```python
from build123d import *

# Parameters (mm, degrees)
BASE_FLANGE1_DEPTH           = 1
EDGE_FLANGE1_STRIP_W         = 8
EDGE_FLANGE1_STRIP_H         = 1
EDGE_FLANGE1_STRIP_CUT_DEPTH = 24
EDGE_FLANGE1_DEPTH           = 24
HEM1_START                   = -12
HEM1_DEPTH                   = 24
HEM1_2_DEPTH                 = 24
CUT_EXTRUDE1_DEPTH           = 10


# Read off the part's stored shape, not the designer's step: Hem1
# Sheet-metal steps are written as plain solids
with BuildPart() as part:
    # Sketch1 → Base-Flange1 (new body)
    with BuildSketch(Plane(origin=(0, 0, 0), x_dir=(1, 0, 0), z_dir=(0, 1, 0))):
        with BuildLine():
            Line((-5.5, 12), (5.5, 12))
            Line((5.5, 12), (18.155635881, 7.546363234))
            ThreePointArc((18.155635881, 7.546363234), (23.5, 0), (18.155635881, -7.546363234))
            Line((18.155635881, -7.546363234), (5.5, -12))
            Line((5.5, -12), (-5.5, -12))
            Line((-5.5, -12), (-5.5, 12))
        make_face()
        with BuildLine():
            Line((10.34, 2.38), (13.012470906, 2.38))
            ThreePointArc((13.012470906, 2.38), (18.942702571, 0), (13.012470906, -2.38))
            Line((13.012470906, -2.38), (10.34, -2.38))
            ThreePointArc((10.34, -2.38), (7.96, 0), (10.34, 2.38))
        make_face(mode=Mode.SUBTRACT)
    extrude(amount=BASE_FLANGE1_DEPTH)

    # Edge-Flange1 strip (across the edge) → Edge-Flange1 strip cut (cut)
    with BuildSketch(Plane(origin=(-5.5, 1, -12), x_dir=(1, 0, 0), z_dir=(0, 0, 1))):
        with Locations((-1, -0.5)):
            Rectangle(EDGE_FLANGE1_STRIP_W, EDGE_FLANGE1_STRIP_H)
    extrude(amount=EDGE_FLANGE1_STRIP_CUT_DEPTH, mode=Mode.SUBTRACT)

    # Edge-Flange1 section (across the edge) → Edge-Flange1 (add)
    with BuildSketch(Plane(origin=(-5.5, 1, -12), x_dir=(1, 0, 0), z_dir=(0, 0, 1))):
        with BuildLine():
            Line((0, 2), (0, 20))
            Line((0, 20), (1, 20))
            Line((1, 20), (1, 2))
            ThreePointArc((1, 2), (1.585786438, 0.585786438), (3, 0))
            Line((3, 0), (3, -1))
            ThreePointArc((3, -1), (0.878679656, -0.121320344), (0, 2))
        make_face()
    extrude(amount=EDGE_FLANGE1_DEPTH)

    # Hem1 outline → Hem1 (cut)
    with BuildSketch(Plane.XY.offset(HEM1_START)):
        with BuildLine():
            ThreePointArc((-5.5, 19.75), (-5.218245837, 20.540569415), (-4.5, 20.974744871))
            Line((-4.5, 20.974744871), (-4.5, 21))
            Line((-4.5, 21), (-5.5, 21))
            Line((-5.5, 21), (-5.5, 19.75))
        make_face()
    extrude(amount=HEM1_DEPTH, mode=Mode.SUBTRACT)

    # Hem1 2 outline → Hem1 2 (add)
    with BuildSketch(Plane.XY.offset(HEM1_START)):
        with BuildLine():
            Line((-4, 17), (-3, 17))
            Line((-3, 17), (-3, 19.75))
            ThreePointArc((-3, 19.75), (-3.459430585, 20.718245837), (-4.5, 20.974744871))
            Line((-4.5, 20.974744871), (-4.5, 19.75))
            ThreePointArc((-4.5, 19.75), (-4.25, 20), (-4, 19.75))
            Line((-4, 19.75), (-4, 17))
        make_face()
    extrude(amount=HEM1_2_DEPTH)

    # Sketch11 → Cut-Extrude1 (cut)
    with BuildSketch(Plane(origin=(-4.5, 0, 0), x_dir=(0, 0, -1), z_dir=(1, 0, 0))):
        with BuildLine():
            Line((-4, 16), (4, 16))
            ThreePointArc((4, 16), (5.414213562, 15.414213562), (6, 14))
            Line((6, 14), (6, 8))
            ThreePointArc((6, 8), (5.414213562, 6.585786438), (4, 6))
            Line((4, 6), (-4, 6))
            ThreePointArc((-4, 6), (-5.414213562, 6.585786438), (-6, 8))
            Line((-6, 8), (-6, 14))
            ThreePointArc((-6, 14), (-5.414213562, 15.414213562), (-4, 16))
        make_face()
    extrude(amount=-CUT_EXTRUDE1_DEPTH, mode=Mode.SUBTRACT)


solid = part.part
```
Here's how the part is built. I have some questions about the finished solid (model axes, mm). A direction names the side the tool comes from. Give positions to 0.01 mm unless a question says otherwise; leave off trailing zeros. Write each loop counter-clockwise with the first axis right and the second up, starting at its lowest first coordinate (ties: lowest second). Pieces come first, ordered by that corner, then holes.
(1) If I drill on L1, parallel to X at y = 19.75, z = 4.75; L2, parallel to Y at x = 11.75, z = 4; L3, parallel to Z at x = 15.5, y = 0.85, over which ranges is the centre line in solid material (lowest first)?
Output values:
L1: x = -5.5 to -4.5, -4 to -3
L2: y = 0 to 1
L3: z = -8.48 to -3.44, 3.44 to 8.48
(2) Imagine slicing it at C-C, the plane x = 15.5. Write out the boundary of the cut face in (y, z), and give its area (3 significant figures).
Output values:
outline: (0, -8.48) - (1, -8.48) - (1, -3.44) - (0, -3.44) - close; (0, 3.44) - (1, 3.44) - (1, 8.48) - (0, 8.48) - close
area: 10.1 mm2
(3) Will these pins go through, and if not, where does the flat tip stop? pin 1 (0.8 mm diameter, centred on x = 12.5, y = 0.5, fed in from -Z); pin 2 (8.5 mm diameter, centred on y = 7.5, z = -1.5, fed in from +X); pin 3 (0.8 mm diameter, centred on y = 18.5, z = -2, fed in from +X); pin 4 (6 mm diameter, centred on y = 3, z = -1, fed in from +X).
Output values:
pin 1: stops at z = -9.68
pin 2: stops at x = -4.5
pin 3: stops at x = -3
pin 4: stops at x = 23.5
(4) On a 3-axis mill with a long thin cutter (end or side, diameter ignored), from which of +Z, -Z, +X, -X, +Y, -Y can I reach the whole of each face in a straight line? I mean faces 5 (the face through (11.7, 0.5, -2.38)), 6 (the face through (-3, 18, 0)), 7 (the face through (-3.5, 17, -0.2)), 8 (the face through (-5, 11, 6)). Say none if no direction works.
Output values:
face 5: +Y, -Y
face 6: +Z, -Z, +X, +Y
face 7: +Z, -Z, +X
face 8: +X, -X
(5) Imagine slicing it at B-B, the plane z = 0. Write out the boundary of the cut face in (x, y), and give its area (3 significant figures).
Output values:
outline: (-5.5, 3) arc R3 ccw to (-2.5, 0) - (7.96, 0) - (7.96, 1) - (-2.5, 1) arc R2 cw to (-4.5, 3) - (-4.5, 6) - (-5.5, 6) - close; (-5.5, 16) - (-4.5, 16) - (-4.5, 19.75) arc R0.25 cw to (-4, 19.75) - (-4, 17) - (-3, 17) - (-3, 19.75) arc R1.25 ccw to (-5.5, 19.75) - close; (18.94, 0) - (23.5, 0) - (23.5, 1) - (18.94, 1) - close
area: 30.8 mm2
(6) Thinking about a two-plate mould opening in Y: for faces 1 (the face through (-4.99, 6.57, 5.4)), 2 (the face through (7.8, 0, -0.2)), 3 (the face through (-3.93, 1.6, -0.17)), 4 (the face through (11.7, 0.5, 2.38)), which applies, pulls with the +Y half, pulls with the -Y half, needs draft (parallel to the pull), parting line crosses it, or undercut?
Output values:
face 1: undercut
face 2: pulls with the -Y half
face 3: undercut
face 4: needs draft
(7) Imagine slicing it at D-D, the plane z = -5.25. Write out the boundary of the cut face in (x, y), and give its area (3 significant figures).
Output values:
outline: (-5.5, 3) arc R3 ccw to (-2.5, 0) - (21.54, 0) - (21.54, 1) - (-2.5, 1) arc R2 cw to (-4.5, 3) - (-4.5, 6.44) - (-5.5, 6.44) - close; (-5.5, 15.56) - (-4.5, 15.56) - (-4.5, 19.75) arc R0.25 cw to (-4, 19.75) - (-4, 17) - (-3, 17) - (-3, 19.75) arc R1.25 ccw to (-5.5, 19.75) - close
area: 40.7 mm2
(8) Imagine slicing it at A-A, the plane y = 11. Write out the boundary of the cut face in (x, z), and give its area (3 significant figures).
Output values:
outline: (-5.5, -12) - (-4.5, -12) - (-4.5, -6) - (-5.5, -6) - close; (-5.5, 6) - (-4.5, 6) - (-4.5, 12) - (-5.5, 12) - close
area: 12.0 mm2
